The model under review builds one solid part; all positions refer to its coordinate system, in mm. Face numbers are marked on the shaded views. A direction names the side the tool comes from. Round coordinates to 2 decimals unless told otherwise and drop trailing zeros. Loops run counter-clockwise (first coordinate to the right, second up) from the corner with the lowest first, then second, coordinate; pieces in that order, holes last. Notation, with made-up numbers: M 67,48 L 107,48 A30 ccw 107,82 Z; hole C 0,-35.5 d11. An arc over 180 degrees is marked long. Use a Markdown table: item, result. Add a question column.
```python
from build123d import *

# Parameters (mm, degrees)
F0_W     = 90.379902
F0_H     = 57.843138
F1_DEPTH = 92.202
F2_R     = 10.424574
F3_T     = -2.54


with BuildPart() as f1:
    # F0 (on Front) → F1 (new body)
    with BuildSketch(Plane.XZ):
        Rectangle(F0_W, F0_H)
    extrude(amount=F1_DEPTH)

    # F2
    f2_edges = [f1.edges().sort_by_distance(p)[0] for p in [
        (45.189951, -92.202, 0),
        (-45.189951, -92.202, 0),
        (45.189951, 0, 0),
        (0, 0, -28.921569),
    ]]
    fillet(f2_edges, radius=F2_R)

    # F3
    f3_openings = [f1.faces().sort_by_distance(p)[0] for p in [
        (-0.120967, -45.977462, 28.921569),
    ]]
    offset(amount=F3_T, openings=f3_openings)


solid = f1.part
```
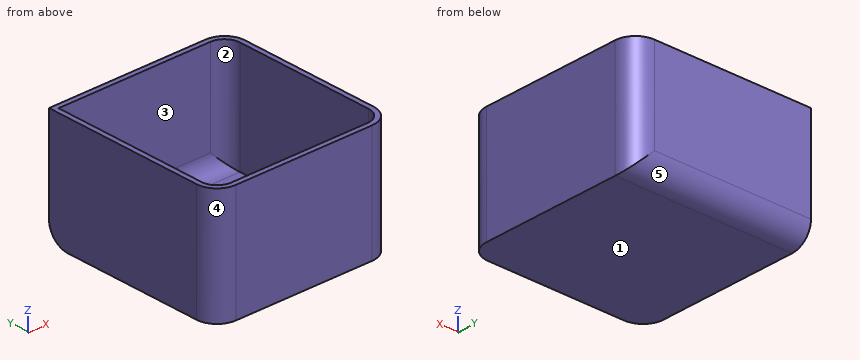
(1) Consider section C-C, the plane y = -15.5. Give the boundary of the cut face in (x, z).
(2) For the marked faces 1 and 2, list the 3-axis set-ups (+Z, -Z, +X, -X, +Y, -Y) from which the entire face can be reached by the end or side of a thin tool; tool diameter is ignored.
(3) Draft analysis for pull direction Y (two halves, no side actions). For the marked faces 3, 4 and 5, state which applies: released by +Y, released by -Y, zero draft, split by the parting line, or undercut.
(4) Consider section A-A, the plane z = 24. Give the boundary of the cut face in (x, y).
(5) Consider section D-D, the plane y = -84. Give the boundary of the cut face in (x, z), then the cut area to 3 significant figures.
(6) Consider section B-B, the plane x = 0. Give the boundary of the cut face in (y, z).
(7) To check wall thickness, follow probe 1 along X at (y, z) = (-11.5, -22.5); probe 2 along Y at (x, z) = (10.5, 15.5); probe 3 along Z at (x, y) = (-16, -34). State the ranges of each line that lie inside material, in increasing order.
(8) Insertion check: pin 1 Ø12 at (x, y) = (4.5, -41.5) entering from +Z. The pin has a flat end and moves straight along its axis. Give the tip position at first contact, or say it passes through.
Found:
| question | item | result |
|---|---|---|
| 1 | outline | M -45.19,-28.92 L 45.19,-28.92 L 45.19,28.92 L 42.65,28.92 L 42.65,-26.38 L -42.65,-26.38 L -42.65,28.92 L -45.19,28.92 Z |
| 2 | face 1 | -Z, +X, -X, +Y, -Y |
| 2 | face 2 | +Z |
| 3 | face 3 | undercut |
| 3 | face 4 | released by -Y |
| 3 | face 5 | released by +Y |
| 4 | outline | M -45.19,-81.78 A10.42 ccw -34.77,-92.2 L 34.77,-92.2 A10.42 ccw 45.19,-81.78 L 45.19,-10.42 A10.42 ccw 34.77,0 L -45.19,0 Z; hole M -42.65,-81.78 A7.88 ccw -34.77,-89.66 L 34.77,-89.66 A7.88 ccw 42.65,-81.78 L 42.65,-10.42 A7.88 ccw 34.77,-2.54 L -42.65,-2.54 Z |
| 5 | outline | M -44.95,-28.92 L 44.95,-28.92 L 44.95,28.92 L 42.33,28.92 L 42.33,-26.38 L -42.33,-26.38 L -42.33,28.92 L -44.95,28.92 Z |
| 5 | area | 518 mm^2 |
| 6 | outline | M -92.2,-28.92 L -10.42,-28.92 A10.42 ccw 0,-18.5 L 0,28.92 L -2.54,28.92 L -2.54,-18.5 A7.88 cw -10.42,-26.38 L -89.66,-26.38 L -89.66,28.92 L -92.2,28.92 Z |
| 7 | probe 1 | x = -45.19 to -42.65, 42.65 to 45.19 |
| 7 | probe 2 | y = -92.2 to -89.66, -2.54 to 0 |
| 7 | probe 3 | z = -28.92 to -26.38 |
| 8 | pin 1 | stops at z = -26.38 |
